Read the model definition and answer for the solid it produces. Units are mm, in the model's axes. Give positions to 0.01 mm unless a question says otherwise; leave off trailing zeros. Loops run counter-clockwise (first coordinate to the right, second up) from the corner with the lowest first, then second, coordinate; pieces in that order, holes last. Notation, with made-up numbers: (-0.75, 64) -> (5.25, 64) arc R12 cw to (5.25, 73) -> close; hole circle Ø5 at (-6.5, -21.5). An arc over 180 degrees is marked (long way). Write each question's results on one line, items separated by ' | '. Start each with the question number.
Item 1: Section B-B on y = -2.5 is taken. State how many separate pieces and enclosed holes the cut face has, and give its area (3 significant figures).
Item 2: Section C-C on z = 12.5 is taken. Write down the section's boundary in (x, y), and give its area (3 significant figures).
Item 3: Each of these flat-tipped pins is pushed along its axis until it touches: P1, Ø2.5, axis at x = -0.5, y = -6, coming from the -Z side; P2, Ø1, axis at y = -6, z = 3.5, coming from the +X side; P3, Ø0.9, axis at x = 0.5, y = -4, coming from the +Z side. Where does it stop, or does it pass through?
Item 4: Find the intervals of material crossed by line 1 (Z direction, x = 0, y = -4); line 2 (X direction, y = -6, z = -6.5); line 3 (X direction, y = -0.75, z = -2.5), in increasing order.
Item 5: Determine the mould class of faces 1 (the cylindrical face through (10, -4, 0)), 2 (the cylindrical face through (-16.39, -4.06, 6.41)), 3 (the flat face through (-96, 0, -10)) for opening direction X: +X half, -X half, draft (parallel to the pull), parting line (faces both ways), or undercut.
Item 6: Section A-A on x = -40 is taken. Write down the section's boundary in (y, z), and give its area (3 significant figures).
Autodesk Inventor part; units mm, degrees
ref_plane "YZ Plane" through (0, 0, 0) normal (1, 0, 0) x (0, 1, 0)
ref_plane "XZ Plane" through (0, 0, 0) normal (0, 1, 0) x (-1, 0, 0)
ref_plane "XY Plane" through (0, 0, 0) normal (0, 0, 1) x (1, 0, 0)
sketch "Sketch1" plane through (0, 0, 0) normal (0, 1, 0) x (-1, 0, 0)
  line L0 (0, 8.5) -> (0, 6.3)
  line L1 (0, -6.3) -> (0, -8.5)
  line L2 (0, 0) -> (150, 0)
  circle A0 centre (150, 0) radius 10
  circle A1 centre (150, 0) radius 15
  circle A2 centre (0, 0) radius 2
  circle A3 centre (0, 0) radius 1.3
  line L3 (0, 1.3) -> (1.5199, 1.3)
  line L4 (0, 1.3) -> (-1.5199, 1.3)
  line L5 (0, -1.3) -> (1.5199, -1.3)
  line L6 (0, -1.3) -> (-1.5199, -1.3)
  circle A4 centre (0, 0) radius 10
  line L7 (0, 10) -> (149.4994, 14.9916)
  line L8 (0, -10) -> (149.4994, -14.9916)
  dimension "d8" = 30
  dimension "d13" = 20
  dimension "d6" = 150
  dimension "d7" = 20
  dimension "d11" = 4
  dimension "d12" = 2.6
extrude "Extrusion2" add sketch "Sketch1" against normal blind 8 contours L4 A2 L3 | L5 A2 L6 | A4 L7 A1 L2 | A4 | L2 A1 L8 A4 | A1
sketch "Sketch3" plane through (0, 0, 0) normal (0, 1, 0) x (1, 0, 0)
  line L0 (-14.4626, 0) -> (-15.2355, -8.0607)
  line L1 (-15.2355, -8.0607) -> (-21.6951, -6.6804)
  line L2 (-21.6951, -6.6804) -> (-37.7613, -6.9565)
  line L3 (-37.7613, -6.9565) -> (-58.9067, -8.8888)
  line L4 (-58.9067, -8.8888) -> (-133.4402, -10.1695)
  line L5 (-133.4402, -10.1695) -> (-129.907, 0)
  line L6 (-129.907, 0) -> (-14.4626, 0)
  line L7 (-14.4626, 0) -> (-15.2355, 8.0607)
  line L8 (-15.2355, 8.0607) -> (-21.6951, 6.6804)
  line L9 (-21.6951, 6.6804) -> (-37.7613, 6.9565)
  line L10 (-37.7613, 6.9565) -> (-58.9067, 8.8888)
  line L11 (-58.9067, 8.8888) -> (-133.4402, 10.1695)
  line L12 (-133.4402, 10.1695) -> (-129.907, 0)
  point P0 (0, 0)
extrude "Extrusion3" cut sketch "Sketch3" against normal through all
fillet "Fillet1" radius 4 12 edges at (-15.2355, -4, -8.0607) (-14.4626, -4, 0) (-15.2355, -4, 8.0607) (-21.6951, -4, 6.6804) (-37.7613, -4, 6.9565) (-21.6951, -4, -6.6804) (-37.7613, -4, -6.9565) (-58.9067, -4, -8.8888) (-133.4402, -4, -10.1695) (-129.907, -4, 0) (-133.4402, -4, 10.1695) (-58.9067, -4, 8.8888)
sketch "Sketch4" plane through (0, 0, 0) normal (0, 1, 0) x (1, 0, 0)
  circle A0 centre (0, 0) radius 6.5
  circle A1 centre (0, 6.5) radius 1.5
  circle A2 centre (0, -6.5) radius 1.5
  dimension "d19" = 13
  dimension "d20" = 3
  dimension "d21" = 3
extrude "Extrusion4" cut sketch "Sketch4" against normal through all contours A1 A0 | A0 A1 | A2 A0 | A0 A2
properties material "Polycarbonate, Clear"
Findings:
1) separate pieces: 1 | enclosed holes: 5 | area: 1,910 mm2
2) outline: (-158.29, -8) -> (-74.88, -8) -> (-74.88, 0) -> (-158.29, 0) -> close | area: 667 mm2
3) P1: z = -10.06 | P2: x = 9.54 | P3: z = 10
4) line 1: -10 to -8, -5 to -1.3, 1.3 to 5, 8 to 10 | line 2: -163.52 to -157.6, -142.4 to -131.76, -16.51 to -1.5, 1.5 to 7.6 | line 3: -164.79 to -159.68, -140.32 to -130.78, -14.7 to 9.68
5) face 1: +X half | face 2: undercut | face 3: draft
6) outline: (-8, -11.34) -> (0, -11.34) -> (0, -7.16) -> (-8, -7.16) -> close; (-8, 7.16) -> (0, 7.16) -> (0, 11.34) -> (-8, 11.34) -> close | area: 66.8 mm2
